For this review, take the finished solid that the model builds, in its own axes (mm). Give positions to 0.01 mm unless a question says otherwise; leave off trailing zeros. Write each loop counter-clockwise with the first axis right and the second up, starting at its lowest first coordinate (ties: lowest second). Pieces come first, ordered by that corner, then holes. Notation, with made-up numbers: M 65.25,24.25 L 80.25,24.25 A18 cw 80.25,43.25 Z; hole C 53.5,7 d8. An arc over 180 degrees is marked long. Use one line per item in the form item = value. Start each with the question number.
Q1. Consider section A-A on x = 0. Write out the cut boundary in (y, z) (1 decimal), and give its area (3 significant figures).
Q2. Clearance check with flat-ended pins moving along their axes: pin 1 Ø1.5 at (x, z) = (-6.5, -11) entering from -Y; pin 2 Ø12 at (x, z) = (-14, 1.5) entering from -Y; pin 3 Ø8 at (y, z) = (-25, -11.5) entering from -X; pin 4 Ø3 at (x, y) = (5, -23.5) entering from -Z (3 decimals). State where each tip first meets the part, or that it passes through.
Q3. Mouldability with a two-part tool opening along Y and no side actions: class faces 1 (the cylindrical face through (-22.37, -17.16, -7.45)), 2 (the cylindrical face through (23.016, 7.248, -5.69)), 3 (the flat face through (-27.32, 7.56, 0)) as released by +Y, released by -Y, zero draft, split by the parting line, or undercut.
Q4. Consider section C-C on z = -10.5. Write out the cut boundary in (x, y).
Q5. For probe 1 along Y at (x, z) = (0, -1.25); probe 2 along X at (y, z) = (-22, 0.25); probe 3 along Y at (x, z) = (-6.5, -7), list the stretches that pass through material, from the lowest coordinate up. Write a range as [from, to].
```python
from build123d import *

# Parameters (mm, degrees)
F0_R     = 28.194
F0_R_2   = 24.13
F1_DEPTH = 15.875
F2_R     = 33.3375
F2_R_2   = 24.13
F3_DEPTH = 4.7625
F4_SIZE  = 0.762


with BuildPart() as f1:
    # F0 (on Top) → F1 (new body)
    with BuildSketch(Plane.XY):
        Circle(F0_R)
        Circle(F0_R_2, mode=Mode.SUBTRACT)
    extrude(amount=-F1_DEPTH)

    # F2 (on Top) → F3 (join)
    with BuildSketch(Plane.XY):
        Circle(F2_R)
        Circle(F2_R_2, mode=Mode.SUBTRACT)
    extrude(amount=F3_DEPTH)

    # F4
    f4_edges = [f1.edges().sort_by_distance(p)[0] for p in [
        (-33.3375, 0, 4.7625),
        (-24.13, 0, 4.7625),
        (-28.194, 0, -15.875),
        (-24.13, 0, -15.875),
    ]]
    chamfer(f4_edges, length=F4_SIZE)


solid = f1.part
```
Working result:
q1.outline = M -33.3,0 L -28.2,0 L -28.2,-15.1 L -27.4,-15.9 L -24.9,-15.9 L -24.1,-15.1 L -24.1,4 L -24.9,4.8 L -32.6,4.8 L -33.3,4 Z; M 24.1,-15.1 L 24.9,-15.9 L 27.4,-15.9 L 28.2,-15.1 L 28.2,0 L 33.3,0 L 33.3,4 L 32.6,4.8 L 24.9,4.8 L 24.1,4 Z
q1.area = 214 mm²
q2.pin_1 = -27.6
q2.pin_2 = -32.36
q2.pin_3 = -18.81
q2.pin_4 = -15.875
q3.face_1 = split by the parting line
q3.face_2 = undercut
q3.face_3 = zero draft
q4.outline = C 0,0 d56.39; hole C 0,0 d48.26
q5.probe_1 = [-28.19, -24.13], [24.13, 28.19]
q5.probe_2 = [-25.05, -9.91], [9.91, 25.05]
q5.probe_3 = [-27.43, -23.24], [23.24, 27.43]
